from build123d import *

# Parameters (mm, degrees)
SKETCH1_W           = 81
SKETCH1_H           = 50
BOSS_EXTRUDE1_DEPTH = 15.5
SKETCH2_W           = 45
SKETCH2_H           = 2.5
CUT_EXTRUDE1_DEPTH  = 51.054969783
FILLET1_R           = 8
FILLET2_R           = 8
FILLET3_R           = 5
FILLET4_R           = 2


with BuildPart() as part:
    # Sketch1 → Boss-Extrude1 (new body)
    with BuildSketch(Plane(origin=(0, 0, 0), x_dir=(1, 0, 0), z_dir=(0, 1, 0))):
        Rectangle(SKETCH1_W, SKETCH1_H)
    extrude(amount=BOSS_EXTRUDE1_DEPTH)

    # Sketch2 → Cut-Extrude1 (cut, through all)
    with BuildSketch(Plane(origin=(0, 15.5, 0), x_dir=(1, 0, 0), z_dir=(0, 1, 0))):
        with Locations((0, 23.75)):
            Rectangle(SKETCH2_W, SKETCH2_H)
        with Locations((0, -23.75)):
            Rectangle(SKETCH2_W, SKETCH2_H)
    extrude(amount=-CUT_EXTRUDE1_DEPTH, mode=Mode.SUBTRACT)

    # Fillet1
    # the kernel refuses this fillet: 8 mm, written as the material it adds along each edge
    with BuildSketch(Plane(origin=(22.5, 15.5, 22.5), x_dir=(-1, 0, 0), z_dir=(0, -1, 0))) as fillet1_piece_1:
        with BuildLine():
            CenterArc((5.809475019, -8), FILLET1_R, 90, 46.567463442)
            Line((0, -2.5), (-0.1161895, -2.39))
            ThreePointArc((-0.1161895, -2.39), (-0.16, -1.25), (-0.16, 0))
            Line((-0.16, 0), (0, 0.16))
            Line((0, 0.16), (5.809475019, 0.16))
            Line((5.809475019, 0.16), (5.809475019, 0))
        make_face()
    extrude(amount=15.5)
    with BuildSketch(Plane(origin=(-22.5, 15.5, 22.5), x_dir=(0, 0, 1), z_dir=(0, -1, 0)), Plane(origin=(22.5, 15.5, -22.5), x_dir=(0, 0, -1), z_dir=(0, -1, 0))) as fillet1_piece_2:
        with BuildLine():
            CenterArc((8, -5.809475019), FILLET1_R, 133.432536558, 46.567463442)
            Line((0, -5.809475019), (-0.16, -5.809475019))
            Line((-0.16, -5.809475019), (-0.16, 0))
            Line((-0.16, 0), (0, 0.16))
            ThreePointArc((0, 0.16), (1.25, 0.16), (2.39, 0.1161895))
            Line((2.39, 0.1161895), (2.5, 0))
        make_face()
    extrude(amount=15.5)
    with BuildSketch(Plane(origin=(-22.5, 15.5, -22.5), x_dir=(0, 0, -1), z_dir=(0, -1, 0))) as fillet1_piece_3:
        with BuildLine():
            CenterArc((8, 5.809475019), FILLET1_R, 180, 46.567463442)
            Line((0, 5.809475019), (-0.16, 5.809475019))
            Line((-0.16, 5.809475019), (-0.16, 0))
            Line((-0.16, 0), (0, -0.16))
            ThreePointArc((0, -0.16), (1.25, -0.16), (2.39, -0.1161895))
            Line((2.39, -0.1161895), (2.5, 0))
        make_face()
    extrude(amount=15.5)

    # Fillet2
    fillet2_edges = [part.edges().sort_by_distance(p)[0] for p in [
        (22.5, 7.75, -25),
        (-22.5, 7.75, -25),
        (22.5, 7.75, 25),
        (-22.5, 7.75, 25),
    ]]
    fillet(fillet2_edges, radius=FILLET2_R)

    # Fillet3
    fillet3_edges = [part.edges().sort_by_distance(p)[0] for p in [
        (-40.5, 7.75, -25),
        (40.5, 7.75, -25),
        (40.5, 7.75, 25),
        (-40.5, 7.75, 25),
    ]]
    fillet(fillet3_edges, radius=FILLET3_R)

    # Fillet4
    fillet4_edges = [part.edges().sort_by_distance(p)[0] for p in [
        (0, 15.5, 22.5),
        (0, 0, 22.5),
        (0, 15.5, -22.5),
        (0, 0, -22.5),
        (18.926592958, 15.5, 22.818854252),
        (-18.926592958, 0, 22.818854252),
        (-18.926592958, 15.5, -22.818854252),
        (18.926592958, 0, -22.818854252),
        (-18.926592958, 15.5, 22.818854252),
        (30.3891535, 15.5, 25),
        (18.926592958, 15.5, -22.818854252),
        (-30.3891535, 15.5, -25),
        (23.042239022, 15.5, 24.681145748),
        (-23.042239022, 15.5, 24.681145748),
        (-23.042239022, 15.5, -24.681145748),
        (23.042239022, 15.5, -24.681145748),
        (30.3891535, 0, 25),
        (18.926592958, 0, 22.818854252),
        (-30.3891535, 0, -25),
        (-18.926592958, 0, -22.818854252),
        (23.042239022, 0, 24.681145748),
        (-23.042239022, 0, 24.681145748),
        (-23.042239022, 0, -24.681145748),
        (23.042239022, 0, -24.681145748),
        (30.3891535, 0, -25),
        (30.3891535, 15.5, -25),
        (40.5, 0, 0),
        (-30.3891535, 0, 25),
        (-40.5, 0, 0),
        (-39.035533906, 0, -23.535533906),
        (-39.035533906, 0, 23.535533906),
        (39.035533906, 0, 23.535533906),
        (39.035533906, 0, -23.535533906),
        (40.5, 15.5, 0),
        (-40.5, 15.5, 0),
        (-30.3891535, 15.5, 25),
        (-39.035533906, 15.5, -23.535533906),
        (-39.035533906, 15.5, 23.535533906),
        (39.035533906, 15.5, 23.535533906),
        (39.035533906, 15.5, -23.535533906),
    ]]
    fillet(fillet4_edges, radius=FILLET4_R)


solid = part.part
Geometry check sheet. Reference: the model listing, model coordinates, mm. A direction names the side the tool comes from. Round coordinates to 2 decimals unless told otherwise and drop trailing zeros. Order: outer loops, then holes, each group sorted by start corner. A loop starts at its lowest first (then second) coordinate and runs counter-clockwise, first axis right, second up. Notation, with made-up numbers: M -26.5,84.25 L -8.5,84.25 A23 cw -8.5,112.25 Z; hole C -30.75,-4 d11. An arc over 180 degrees is marked long. Answer in a Markdown table with one row per item. Add a question column.
Item 1: Material ranges on L1, parallel to Z at x = -4, y = 6; L2, parallel to Z at x = 25, y = 14.75; L3, parallel to X at y = 2, z = 22, recorded low to high. Write a range as [from, to].
Item 2: Sectioned sample at B-B, the plane y = 3. Enter the section's corners in (x, z), plus the area to 3 significant figures.
Item 3: Sectioned sample at A-A, the plane x = -3. Enter the section's corners in (y, z).
Item 4: Set-up check for faces 1 (the face through (0, 8, 22.5)), 2 (the face through (0.23, 0.6, 21.93)), 3 (the face through (0, 8, -22.5)): record each of +Z, -Z, +X, -X, +Y, -Y from which the full face is reachable in a straight line by a thin tool's end or side.
Item 5: Depth check by flat-ended pin: pin 1 Ø6 at (x, y) = (-13, 6.5) entering from +Z; pin 2 Ø9 at (x, y) = (-3.5, 6) entering from -Z. Enter the tip coordinate at first touch or a pass-through.
Item 6: Draft check along X on faces 4 (the face through (39.93, 0.6, -0.28)), 5 (the face through (-39.93, 0.6, 0.28)), 6 (the face through (-0.23, 0.6, -21.93)), 7 (the face through (30, 8, 25)). Enter one of: released by +X, released by -X, zero draft, split by the parting line, or undercut.
Filled in:
| question | item | result |
|---|---|---|
| 1 | L1 | z = [-22.5, 22.5] |
| 1 | L2 | z = [-24.56, 24.56] |
| 1 | L3 | x = [-40.08, 40.08] |
| 2 | outline | M -40.5,-20 A5 ccw -35.5,-25 L -25.28,-25 A8 ccw -20.98,-23.75 A8 cw -16.69,-22.5 L 16.69,-22.5 A8 cw 20.98,-23.75 A8 ccw 25.28,-25 L 35.5,-25 A5 ccw 40.5,-20 L 40.5,20 A5 ccw 35.5,25 L 25.28,25 A8 ccw 20.98,23.75 A8 cw 16.69,22.5 L -16.69,22.5 A8 cw -20.98,23.75 A8 ccw -25.28,25 L -35.5,25 A5 ccw -40.5,20 Z |
| 2 | area | 3,820 mm² |
| 3 | outline | M 0,-20.5 A2 ccw 2,-22.5 L 13.5,-22.5 A2 ccw 15.5,-20.5 L 15.5,20.5 A2 ccw 13.5,22.5 L 2,22.5 A2 ccw 0,20.5 Z |
| 4 | face 1 | +Z, +Y, -Y |
| 4 | face 2 | +Z, -Y |
| 4 | face 3 | -Z, +Y, -Y |
| 5 | pin 1 | stops at z = 22.5 |
| 5 | pin 2 | stops at z = -22.5 |
| 6 | face 4 | released by +X |
| 6 | face 5 | released by -X |
| 6 | face 6 | undercut |
| 6 | face 7 | zero draft |
